Could you check a few things on this drawing? It's one solid part, dimensions in mm from its lowest x, y, z. A direction names the side the tool comes from. Coordinates: 2 decimals unless noted, no trailing zeros. Loops run counter-clockwise (first coordinate to the right, second up) from the corner with the lowest first, then second, coordinate; pieces in that order, holes last. Notation, with made-up numbers: M 62,44.25 L 107,44.25 A5 cw 107,49.25 Z; hole C -14,-10 d6. An arc over 180 degrees is marked long. Answer as a JSON object with one key per item and string values. Group by question number.
Item 1: Suppose I cut it at A-A (z = 2). Write out the boundary of the cut face in (x, y), then the cut area to 3 significant figures.
Item 2: Suppose I cut it at C-C (z = 5). Write out the boundary of the cut face in (x, y), then the cut area to 4 significant figures.
Item 3: Suppose I cut it at D-D (y = 11). Write out the boundary of the cut face in (x, z).
Item 4: Suppose I cut it at B-B (x = 5). Write out the boundary of the cut face in (y, z).
Item 5: If I drill on line 1 (Y direction, x = 4.5, z = 2.25); line 2 (Y direction, x = 4.5, z = 3.75); line 3 (Z direction, x = 6.5, y = 6), over which ranges is the centre line in solid material (lowest first)?
Item 6: We'd pull the mould along X, two halves only. Please class the marked faces 3, 4 and 5: +X half, -X half, draft (parallel to the pull), parting line (faces both ways), or undercut.
Item 7: I'm going to push flat-ended pins straight in: pin 1 Ø2 at (x, y) = (7, 7.5) entering from +Z; pin 2 Ø5 at (x, z) = (3.5, 4.5) entering from -Y; pin 3 Ø2 at (x, y) = (7.5, 9) entering from -Z; pin 4 Ø4 at (x, y) = (6, 10.5) entering from +Z. Where does each tip first touch, or does it pass through?
Item 8: Which directions (+Z, -Z, +X, -X, +Y, -Y) give clear straight access to the entire face, cutting with the end or side of a thin tool? Please do the marked faces 1 and 2.
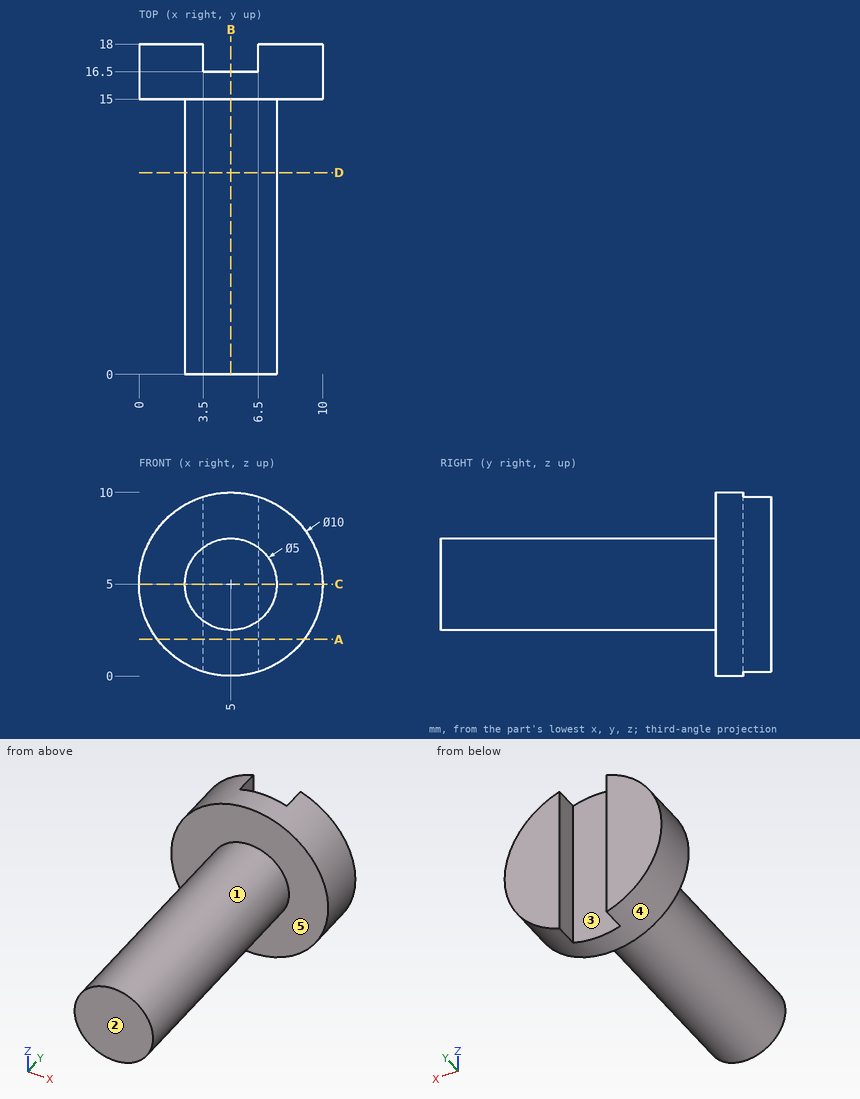
From the geometry:
{
 "1": {"outline": "M 1,15 L 9,15 L 9,18 L 6.5,18 L 6.5,16.5 L 3.5,16.5 L 3.5,18 L 1,18 Z", "area": "19.5 mm2"},
 "2": {"outline": "M 0,15 L 2.5,15 L 2.5,0 L 7.5,0 L 7.5,15 L 10,15 L 10,18 L 6.5,18 L 6.5,16.5 L 3.5,16.5 L 3.5,18 L 0,18 Z", "area": "100.5 mm2"},
 "3": {"outline": "C 5,5 d5"},
 "4": {"outline": "M 0,2.5 L 15,2.5 L 15,0 L 16.5,0 L 16.5,10 L 15,10 L 15,7.5 L 0,7.5 Z"},
 "5": {"line 1": "15 to 16.5", "line 2": "0 to 16.5", "line 3": "3 to 7"},
 "6": {"face 3": "undercut", "face 4": "parting line", "face 5": "draft"},
 "7": {"pin 1": "z = 7.29", "pin 2": "y = 0", "pin 3": "z = 3", "pin 4": "z = 7.5"},
 "8": {"face 1": "-Y", "face 2": "+Z, -Z, +X, -X, -Y"}
}
